Design review of the part built by this model. Coordinates are the model's own, in mm. Coordinates: 2 decimals unless noted, no trailing zeros. Loops run counter-clockwise (first coordinate to the right, second up) from the corner with the lowest first, then second, coordinate; pieces in that order, holes last. Notation, with made-up numbers: (83, 22.25) -> (106, 22.25) arc R27 cw to (106, 61.25) -> close; hole circle Ø4 at (36.5, 0). An arc over 180 degrees is marked (long way). Use CSV: the item, a comma, the result in double quotes.
```python
from build123d import *

# Parameters (mm, degrees)
BOSS_EXTRUDE1_DEPTH = 4.5
SKETCH2_W           = 0.25
SKETCH2_H           = 0.25
BOSS_EXTRUDE2_DEPTH = 14.5


with BuildPart() as part:
    # Sketch1 → Boss-Extrude1 (new body)
    with BuildSketch(Plane(origin=(0, 0, 0), x_dir=(1, 0, 0), z_dir=(0, 1, 0))):
        with BuildLine():
            Line((0, 0), (4.3, 0))
            ThreePointArc((4.3, 0), (2.15, -3.2), (0, 0))
        make_face()
    extrude(amount=BOSS_EXTRUDE1_DEPTH)

    # Sketch2 → Boss-Extrude2 (add)
    with BuildSketch(Plane(origin=(0, 4.5, 0), x_dir=(1, 0, 0), z_dir=(0, 1, 0))):
        with Locations((3.3, -1.125)):
            Rectangle(SKETCH2_W, SKETCH2_H)
        with Locations((2.15, -1.125)):
            Rectangle(SKETCH2_W, SKETCH2_H)
        with Locations((1, -1.125)):
            Rectangle(SKETCH2_W, SKETCH2_H)
    extrude(amount=BOSS_EXTRUDE2_DEPTH)


solid = part.part
```
Item 1: Clearance check with flat-ended pins moving along their axes: pin 1 (1 mm diameter, centred on x = 3.5, y = 7, fed in from -Z); pin 2 (1.5 mm diameter, centred on x = 3, y = 6.5, fed in from +Z); pin 3 (1 mm diameter, centred on y = 9, z = 1.5, fed in from +X) (3 decimals). State where each tip first meets the part, or that it passes through.
Checked values:
pin 1,"z = 1"
pin 2,"z = 1.25"
pin 3,"x = 3.425"
Item 2: To check wall thickness, follow line 1 along X through (y, z) = (16.25, 1.2) (3 decimals); line 2 along Y through (x, z) = (3.95, 1.3); line 3 along Z through (x, y) = (2.2, 6). State the ranges of each line that lie inside material, in increasing order.
Checked values:
line 1,"0.875 to 1.125, 2.025 to 2.275, 3.175 to 3.425"
line 2,"0 to 4.5"
line 3,"1 to 1.25"
Item 3: Add section C-C (x = 4.1). Give the boundary of the cut face in (y, z), then the cut area to 3 significant figures.
Checked values:
outline,"(0, 0) -> (4.5, 0) -> (4.5, 2.14) -> (0, 2.14) -> close"
area,"9.62 mm^2"
Item 4: Add section A-A (y = 8.75). Give the boundary of the cut face in (x, z) (3 decimals).
Checked values:
outline,"(0.875, 1) -> (1.125, 1) -> (1.125, 1.25) -> (0.875, 1.25) -> close; (2.025, 1) -> (2.275, 1) -> (2.275, 1.25) -> (2.025, 1.25) -> close; (3.175, 1) -> (3.425, 1) -> (3.425, 1.25) -> (3.175, 1.25) -> close"
Item 5: Add section D-D (y = 3). Give the boundary of the cut face in (x, z).
Checked values:
outline,"(0, 0) -> (4.3, 0) arc R2.32 ccw (long way) to start"
Item 6: Add section B-B (z = 0.35). Give the boundary of the cut face in (x, y).
Checked values:
outline,"(-0.11, 0) -> (4.41, 0) -> (4.41, 4.5) -> (-0.11, 4.5) -> close"
